from build123d import *

# Parameters (mm, degrees)
F0_W     = 63.5
F0_H     = 21.427987
F1_DEPTH = 3.175
F2_DEPTH = 25.4
F0_H_2   = 7.839117
F3_DEPTH = 12.7
F0_H_3   = 88.9
F4_DEPTH = 3.175


with BuildPart() as f1:
    # F0 (on Top) → F1 (new body)
    with BuildSketch(Plane.XY):
        with Locations((0, -63.00311)):
            Rectangle(F0_W, F0_H)
    extrude(amount=F1_DEPTH)

    # F0 (on Top) → F2 (join)
    with BuildSketch(Plane.XY):
        Polygon((-31.75, 44.45), (31.75, 44.45), (31.75, -44.45), (31.75, -52.289117), (31.75, -73.717104), (38.1, -73.717104), (38.1, 53.282896), (-38.1, 53.282896), (-38.1, -73.717104), (-31.75, -73.717104), (-31.75, -52.289117), (-31.75, -44.45), align=None)
    extrude(amount=F2_DEPTH)

    # F0 (on Top) → F3 (join)
    with BuildSketch(Plane.XY):
        with Locations((0, -48.369558)):
            Rectangle(F0_W, F0_H_2)
    extrude(amount=F3_DEPTH)

    # F0 (on Top) → F4 (join)
    with BuildSketch(Plane.XY):
        Rectangle(F0_W, F0_H_3)
    extrude(amount=F4_DEPTH)


solid = f1.part
Work out the finished part from the listing and answer in its coordinate system (mm). A direction names the side the tool comes from. Give positions to 0.01 mm unless a question says otherwise; leave off trailing zeros. Loops run counter-clockwise (first coordinate to the right, second up) from the corner with the lowest first, then second, coordinate; pieces in that order, holes last. Notation, with made-up numbers: (16.25, 57.25) - (48.25, 57.25) arc R18 ccw to (48.25, 64.25) - close; hole circle Ø5 at (6, 19). An arc over 180 degrees is marked (long way). Answer in a Markdown table with one row per item.
(1) Section D-D (z = 15) is taken. Give the vertices of the cut face in (x, y).
Results list:
| item | result |
|---|---|
| outline | (-38.1, -73.72) - (-31.75, -73.72) - (-31.75, 44.45) - (31.75, 44.45) - (31.75, -73.72) - (38.1, -73.72) - (38.1, 53.28) - (-38.1, 53.28) - close |
(2) Section A-A (y = 23) is taken. Give the vertices of the cut face in (x, z) (3 decimals), and give its area (3 significant figures).
Results list:
| item | result |
|---|---|
| outline | (-38.1, 0) - (38.1, 0) - (38.1, 25.4) - (31.75, 25.4) - (31.75, 3.175) - (-31.75, 3.175) - (-31.75, 25.4) - (-38.1, 25.4) - close |
| area | 524 mm² |
(3) Section C-C (x = -16) is taken. Give the vertices of the cut face in (y, z) (3 decimals).
Results list:
| item | result |
|---|---|
| outline | (-73.717, 0) - (53.283, 0) - (53.283, 25.4) - (44.45, 25.4) - (44.45, 3.175) - (-44.45, 3.175) - (-44.45, 12.7) - (-52.289, 12.7) - (-52.289, 3.175) - (-73.717, 3.175) - close |
(4) A tool of negligible diameter and unlimited length cuts with its end or side. For faces 1 (the face through (0, -63, 3.175)), 2 (the face through (35, -73.717, 13)), 3 (the face through (0, 44.45, 14)), from which of +Z, -Z, +X, -X, +Y, -Y can it reach the whole face along a straight path? Write none if from no direction.
Results list:
| item | result |
|---|---|
| face 1 | +Z, -Y |
| face 2 | +Z, -Z, +X, -X, -Y |
| face 3 | +Z |
(5) For a pull along Y with two mould halves and no side action, classify faces 4 (the face through (0, -73.717, 2)), 5 (the face through (0, 1, 3.175)), 6 (the face through (-38.1, -9, 13)) as pulls with the +Y half, pulls with the -Y half, needs draft (parallel to the pull), parting line crosses it, or undercut.
Results list:
| item | result |
|---|---|
| face 4 | pulls with the -Y half |
| face 5 | undercut |
| face 6 | needs draft |
(6) Flat-ended cylindrical pins translate along their axes: pin 1 Ø6 at (x, z) = (16, 19) entering from -Y; pin 2 Ø6 at (x, z) = (-6.5, 9.5) entering from -Y; pin 3 Ø6.5 at (x, y) = (2, -63.5) entering from +Z (3 decimals). Find the tip coordinate at first contact, or state that the pin passes through.
Results list:
| item | result |
|---|---|
| pin 1 | stops at y = 44.45 |
| pin 2 | stops at y = -52.29 |
| pin 3 | stops at z = 3.175 |
(7) Consider L1, parallel to X at y = -21, z = 16; L2, parallel to Y at x = 6.5, z = 12; L3, parallel to Y at x = 26, z = 17. Determine where each line is inside the solid, lowest interval first. Write a range as [from, to].
Results list:
| item | result |
|---|---|
| L1 | x = [-38.1, -31.75], [31.75, 38.1] |
| L2 | y = [-52.29, -44.45], [44.45, 53.28] |
| L3 | y = [44.45, 53.28] |
(8) Section B-B (z = 6) is taken. Give the vertices of the cut face in (x, y).
Results list:
| item | result |
|---|---|
| outline | (-38.1, -73.72) - (-31.75, -73.72) - (-31.75, -52.29) - (31.75, -52.29) - (31.75, -73.72) - (38.1, -73.72) - (38.1, 53.28) - (-38.1, 53.28) - close; hole (-31.75, -44.45) - (31.75, -44.45) - (31.75, 44.45) - (-31.75, 44.45) - close |
